The listing builds one solid part. Answer for the finished solid, in the listing's coordinates (mm). Face numbers are marked on the shaded views. A direction names the side the tool comes from. Give positions to 0.01 mm unless a question says otherwise; leave off trailing zeros. Loops run counter-clockwise (first coordinate to the right, second up) from the corner with the lowest first, then second, coordinate; pieces in that order, holes last. Notation, with made-up numbers: M -3.5,22 L 47.5,22 A26 ccw 47.5,47 Z; hole C 6,29.5 d3. An arc over 180 degrees is marked long. Use one line per item in the form item = value. Start each with the question number.
1. The part is cut by section A-A (y = 438.5). Write down the section's boundary in (x, z), and give its area (3 significant figures).
2. The part is cut by section B-B (x = 584). Write down the section's boundary in (y, z).
3. Straight lines are drawn through the part: line 1 (X direction, y = 1.5, z = 35.5); line 2 (Z direction, x = -123, y = 165); line 3 (Y direction, x = 209, z = 41). For each, find the intervals that lie inside material, in ascending order. Write a range as from..to.
4. The part is cut by section C-C (z = 156). Write down the section's boundary in (x, y), and give its area (3 significant figures).
5. For the marked faces 4 and 5, determine the directions among +Z, -Z, +X, -X, +Y, -Y from which every point of the face is accessible in a straight line to the end or side of a thin tool.
6. The mould has two halves that part along X. Classify the marked faces 1, 2 and 3: released by +X, released by -X, zero draft, split by the parting line, or undercut.
7. Each of these flat-tipped pins is pushed along its axis until it touches: pin 1 Ø1 at (x, z) = (-146.5, 133.5) entering from -Y; pin 2 Ø4 at (x, y) = (116, -99.5) entering from -Z. Where does it stop, or does it pass through?
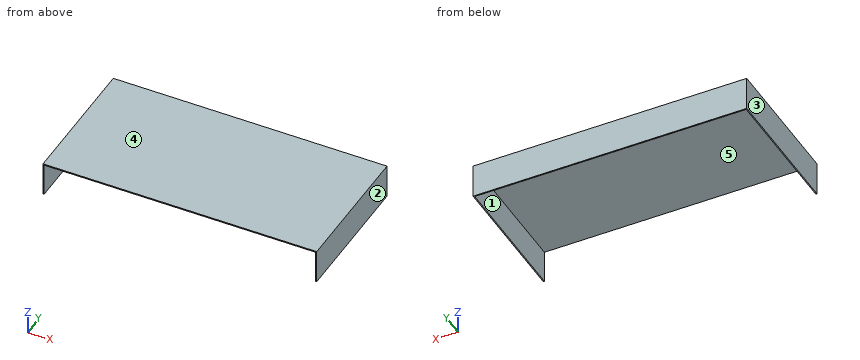
from build123d import *

# Parameters (mm, degrees)
F0_W     = 1524
F0_H     = 762
F1_DEPTH = 190.5
F2_T     = -6.35
F3_W     = 1511.3
F3_H     = 184.15
F4_DEPTH = 25.4


with BuildPart() as f1:
    # F0 (on Top) → F1 (new body)
    with BuildSketch(Plane.XY):
        with Locations((41.196167, 129.838063)):
            Rectangle(F0_W, F0_H)
    extrude(amount=F1_DEPTH)

    # F2
    f2_openings = [f1.faces().sort_by_distance(p)[0] for p in [
        (41.196167, 129.838063, 0),
    ]]
    offset(amount=F2_T, openings=f2_openings)

    # F3 (on face) → F4 (cut)
    with BuildSketch(Plane(origin=(0, -244.811937, 0), x_dir=(-1, 0, 0), z_dir=(0, 1, 0))):
        with Locations((-41.196167, 92.075)):
            Rectangle(F3_W, F3_H)
    extrude(amount=-F4_DEPTH, mode=Mode.SUBTRACT)


solid = f1.part
Derived:
q1.outline = M -720.8,0 L -714.45,0 L -714.45,184.15 L 796.85,184.15 L 796.85,0 L 803.2,0 L 803.2,190.5 L -720.8,190.5 Z
q1.area = 12,000 mm2
q2.outline = M -251.16,184.15 L 504.49,184.15 L 504.49,0 L 510.84,0 L 510.84,190.5 L -251.16,190.5 Z
q3.line_1 = -720.8..-714.45, 796.85..803.2
q3.line_2 = 184.15..190.5
q3.line_3 = 504.49..510.84
q4.outline = M -720.8,-251.16 L -714.45,-251.16 L -714.45,504.49 L 796.85,504.49 L 796.85,-251.16 L 803.2,-251.16 L 803.2,510.84 L -720.8,510.84 Z
q4.area = 19,300 mm2
q5.face_4 = +Z, +X, -X, +Y, -Y
q5.face_5 = -Z, -Y
q6.face_1 = undercut
q6.face_2 = released by +X
q6.face_3 = released by -X
q7.pin_1 = 504.49
q7.pin_2 = 184.15
